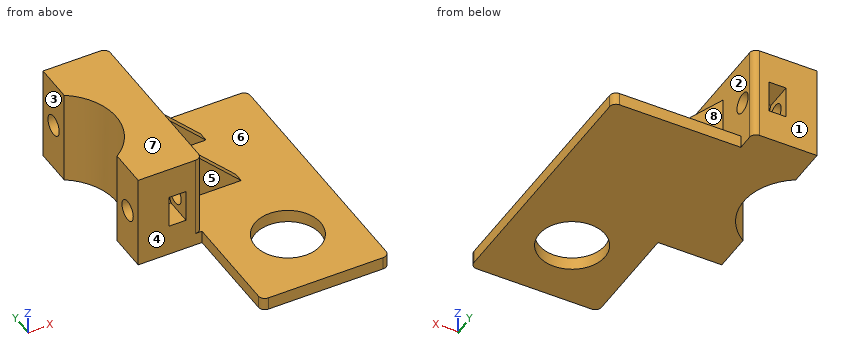
from build123d import *

# Parameters (mm, degrees)
CYLINDER_R               = 3.2
CYLINDER_DEPTH           = 30
EXTRUDE004_DEPTH         = 5.3
CLONE002_PLACEMENT_ANGLE = 180
EXTRUDE002_DEPTH         = 30
EXTRUDE003_DEPTH         = 3
SKETCH_R                 = 10.3
EXTRUDE_DEPTH            = 4
FILLET_R                 = 2


with BuildPart() as bohrung:
    # Cylinder → Cylinder (new body)
    with BuildSketch(Plane(origin=(0, -21, 15), x_dir=(0, 0, 1), z_dir=(-1, 0, 0))):
        Circle(CYLINDER_R)
    extrude(amount=CYLINDER_DEPTH)


with BuildPart() as bohrung001:
    # Clone base: copy of Bohrung
    add(bohrung.part)


with BuildPart() as bohrung001_1:
    # Clone placement: moved
    add(bohrung001.part.moved(Location((0, 42, 0))))


with BuildPart() as obj1:
    # Sketch004 → Extrude004 (new body)
    with BuildSketch(Plane(origin=(0, 0, 0), x_dir=(0, -1, 0), z_dir=(-1, 0, 0))):
        Polygon((15.5, 15), (18.444486, 20.1), (30.444486, 20.1), (30.444486, 9.9), (18.444486, 9.9), align=None)
    extrude(amount=EXTRUDE004_DEPTH)


with BuildPart() as obj1_1:
    # Extrude004 placement: moved
    add(obj1.part.moved(Location((-5, 0, 0))))


with BuildPart() as obj2:
    # Clone002 base: copy of obj1
    add(obj1_1.part)


with BuildPart() as obj2_1:
    # Clone002 placement: moved
    add(obj2.part.moved(Location((0, 0, 30))).rotate(Axis((0, 0, 30), (1, 0, 0)), CLONE002_PLACEMENT_ANGLE))


with BuildPart() as obj3:
    # Fusion base: copy of Bohrung
    add(bohrung.part)

    # Fusion: union Bohrung001, obj2, obj1
    add(bohrung001_1.part)
    add(obj2_1.part)
    add(obj1_1.part)


with BuildPart() as obj4:
    # Sketch002 → Extrude002 (new body)
    with BuildSketch(Plane.XY):
        with BuildLine():
            Line((-20, 27), (0, 27))
            Line((0, 27), (0, -27))
            Line((0, -27), (-20, -27))
            Line((-20, -27), (-20, -15))
            ThreePointArc((-20, -15), (-11.949874, 0), (-20, 15))
            Line((-20, 15), (-20, 27))
        make_face()
    extrude(amount=EXTRUDE002_DEPTH)


with BuildPart() as winkel:
    # Sketch003 → Extrude003 (new body)
    with BuildSketch(Plane.XZ):
        Polygon((0, 24), (20, 4), (0, 4), align=None)
    extrude(amount=EXTRUDE003_DEPTH)


with BuildPart() as winkel_1:
    # Extrude003 placement: moved
    add(winkel.part.moved(Location((0, -10, 0))))


with BuildPart() as winkel001:
    # Clone001 base: copy of Winkel
    add(winkel_1.part)


with BuildPart() as winkel001_1:
    # Clone001 placement: moved
    add(winkel001.part.moved(Location((0, 20, 0))))


with BuildPart() as obj5:
    # Sketch → Extrude (new body)
    with BuildSketch(Plane.XY):
        with BuildLine():
            Line((38, 0), (2, 0))
            ThreePointArc((0, 2), (0.585786, 0.585786), (2, 0))
            Line((0, 2), (0, 81))
            Line((0, 81), (38, 81))
            ThreePointArc((40, 79), (39.414214, 80.414214), (38, 81))
            Line((40, 79), (40, 2))
            ThreePointArc((38, 0), (39.414214, 0.585786), (40, 2))
        make_face()
        with Locations((20, 21.5)):
            Circle(SKETCH_R, mode=Mode.SUBTRACT)
    extrude(amount=EXTRUDE_DEPTH)


with BuildPart() as obj5_1:
    # Extrude placement: moved
    add(obj5.part.moved(Location((0, -61, 0))))

    # Fusion001: union obj4, Winkel, Winkel001
    add(obj4.part)
    add(winkel_1.part)
    add(winkel001_1.part)

    # Fillet
    fillet_edges = [obj5_1.edges().sort_by_distance(p)[0] for p in [
        (0, -27, 17),
        (0, 27, 15),
    ]]
    fillet(fillet_edges, radius=FILLET_R)

    # Cut: cut obj3
    add(obj3.part, mode=Mode.SUBTRACT)


solid = obj5_1.part
Read the model definition and answer for the solid it produces. Units are mm, in the model's axes. Face numbers are marked on the shaded views. A direction names the side the tool comes from. Give positions to 0.01 mm unless a question says otherwise; leave off trailing zeros. Write each loop counter-clockwise with the first axis right and the second up, starting at its lowest first coordinate (ties: lowest second). Pieces come first, ordered by that corner, then holes. Notation, with made-up numbers: (16.25, 42) - (40.25, 42) arc R22 ccw to (40.25, 66) - close; hole circle Ø8 at (-9, 62.25). An arc over 180 degrees is marked (long way). Answer in a Markdown table with one row per item. Add a question column.
Item 1: A tool of negligible diameter and unlimited length cuts with its end or side. For the marked faces 4, 5, 6, 7 and 8, from which of +Z, -Z, +X, -X, +Y, -Y can it reach the whole face along a straight path? Write none if from no direction.
Item 2: Section C-C, the plane x = 26 is taken. Write down the section's boundary in (y, z), and give its area (3 significant figures).
Item 3: Section A-A, the plane y = 21 is taken. Write down the section's boundary in (x, z), and give its area (3 significant figures).
Item 4: Find the intervals of material crossed by L1, parallel to Y at x = -3.8, z = 15; L2, parallel to Z at x = -3.7, y = -21; L3, parallel to Y at x = 13.5, z = 5, in increasing order.
Item 5: Section D-D, the plane z = 26.5 is taken. Write down the section's boundary in (x, y).
Item 6: Determine the mould class of the marked faces 1, 2 and 3 for opening direction Y: pulls with the +Y half, pulls with the -Y half, needs draft (parallel to the pull), parting line crosses it, or undercut.
Item 7: Flat-ended cylindrical pins translate along their axes: P1, Ø6, axis at x = -9, z = 9, coming from the -Y side; P2, Ø6, axis at y = -21, z = 15, coming from the -X side; P3, Ø12.5, axis at x = 24.5, y = -2.5, coming from the +Z side; P4, Ø1.2, axis at x = 12.5, z = 2.5, coming from the +Y side. Find the tip coordinate at first contact, or state that the pin passes through.
Item 8: Section B-B, the plane z = 2.5 is taken. Write down the section's boundary in (x, y), and give its area (3 significant figures).
Recorded:
| question | item | result |
|---|---|---|
| 1 | face 4 | +Z, -Z, -X, -Y |
| 1 | face 5 | +Z, +X, -Y |
| 1 | face 6 | +Z, +X |
| 1 | face 7 | +Z, +X, -X, +Y, -Y |
| 1 | face 8 | +Z, +X, +Y |
| 2 | outline | (-61, 0) - (-47.87, 0) - (-47.87, 4) - (-61, 4) - close; (-31.13, 0) - (20, 0) - (20, 4) - (-31.13, 4) - close |
| 2 | area | 257 mm2 |
| 3 | outline | (-20, 0) - (0, 0) - (0, 11.8) - (-5, 11.8) - (-5, 9.9) - (-10.3, 9.9) - (-10.3, 11.8) - (-20, 11.8) - close; (-20, 18.2) - (-10.3, 18.2) - (-10.3, 20.1) - (-5, 20.1) - (-5, 18.2) - (0, 18.2) - (0, 30) - (-20, 30) - close |
| 3 | area | 452 mm2 |
| 4 | L1 | y = -27 to -24.2, -17.8 to 17.8, 24.2 to 27 |
| 4 | L2 | z = 0 to 11.8, 18.2 to 30 |
| 4 | L3 | y = -13 to -10, 7 to 10 |
| 5 | outline | (-20, -27) - (-2, -27) arc R2 ccw to (0, -25) - (0, 25) arc R2 ccw to (-2, 27) - (-20, 27) - (-20, 15) arc R18 cw to (-20, -15) - close |
| 6 | face 1 | pulls with the +Y half |
| 6 | face 2 | undercut |
| 6 | face 3 | needs draft |
| 7 | P1 | stops at y = -27 |
| 7 | P2 | passes through |
| 7 | P3 | stops at z = 4 |
| 7 | P4 | stops at y = 20 |
| 8 | outline | (-20, -27) - (0, -27) - (0, -59) arc R2 ccw to (2, -61) - (38, -61) arc R2 ccw to (40, -59) - (40, 18) arc R2 ccw to (38, 20) - (0, 20) - (0, 25) arc R2 ccw to (-2, 27) - (-20, 27) - (-20, 15) arc R18 cw to (-20, -15) - close; hole circle Ø20.6 at (20, -39.5) |
| 8 | area | 3,810 mm2 |
